Source: CAD feature listing. Evaluate the final solid. Frame: model axes, mm. Coordinates: 2 decimals unless noted, no trailing zeros. Loops run counter-clockwise (first coordinate to the right, second up) from the corner with the lowest first, then second, coordinate; pieces in that order, holes last. Notation, with made-up numbers: M 25,6 L 57,6 A17 cw 57,15 Z; hole C -27,5.25 d5. An arc over 180 degrees is marked long. Write each question's results on one line, items separated by ' | '. Start each with the question number.
from build123d import *

# Parameters (mm, degrees)
SKETCH_W        = 55
SKETCH_H        = 55
SKETCH_R        = 1.5
SKETCH_R_2      = 2.75
PAD_DEPTH       = 5
SKETCH001_R     = 4.5
POCKET_DEPTH    = 2
SKETCH002_R     = 3
POCKET001_DEPTH = 2


with BuildPart() as part:
    # Sketch → Pad (new body)
    with BuildSketch(Plane.XY):
        with Locations((27.5, 27.5)):
            Rectangle(SKETCH_W, SKETCH_H)
        with Locations((7.5, 47.5)):
            Circle(SKETCH_R, mode=Mode.SUBTRACT)
        with Locations((47.5, 7.5)):
            Circle(SKETCH_R, mode=Mode.SUBTRACT)
        with Locations((40, 40)):
            Circle(SKETCH_R_2, mode=Mode.SUBTRACT)
        with Locations((15, 15)):
            Circle(SKETCH_R_2, mode=Mode.SUBTRACT)
    extrude(amount=PAD_DEPTH)

    # Sketch001 → Pocket (cut)
    with BuildSketch(Plane.XY.offset(5)):
        with Locations((40, 40)):
            Circle(SKETCH001_R)
        with Locations((15, 15)):
            Circle(SKETCH001_R)
    extrude(amount=-POCKET_DEPTH, mode=Mode.SUBTRACT)

    # Sketch002 → Pocket001 (cut)
    with BuildSketch(Plane(origin=(0, 0, 0), x_dir=(1, 0, 0), z_dir=(0, 0, -1))):
        with Locations((47.5, -7.5)):
            Circle(SKETCH002_R)
        with Locations((7.5, -47.5)):
            Circle(SKETCH002_R)
    extrude(amount=-POCKET001_DEPTH, mode=Mode.SUBTRACT)


solid = part.part
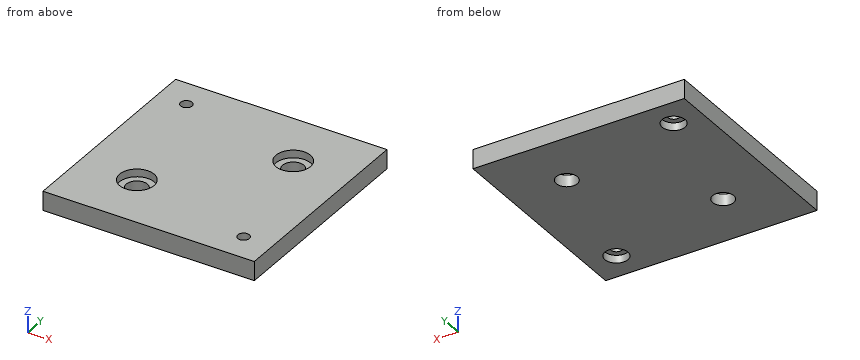
Item 1: Cut plane C-C (z = 1.3). Output: boundary loops of the cut face in (x, y).
Item 2: Cut plane A-A (x = 47.5). Output: boundary loops of the cut face in (y, z).
Item 3: Line query: probe 1 along X at (y, z) = (47.5, 1.05); probe 2 along Y at (x, z) = (40, 3.55); probe 3 along X at (y, z) = (47.5, 3.9). Output: solid intervals per line, ascending.
Item 4: Cut plane B-B (y = 40). Output: boundary loops of the cut face in (x, z).
Item 5: Cut plane D-D (x = 18.5). Output: boundary loops of the cut face in (y, z), then the cut area to 3 significant figures.
Item 6: First-contact query: pin 1 Ø8 at (x, y) = (40, 40) entering from +Z; pin 2 Ø3.5 at (x, y) = (7.5, 47.5) entering from -Z. Flat tips, straight axial feed; report the tip coordinate or a pass-through.
Response values:
1) outline: M 0,0 L 55,0 L 55,55 L 0,55 Z; hole C 7.5,47.5 d6; hole C 15,15 d5.5; hole C 40,40 d5.5; hole C 47.5,7.5 d6
2) outline: M 0,0 L 4.5,0 L 4.5,2 L 6,2 L 6,5 L 0,5 Z; M 9,2 L 10.5,2 L 10.5,0 L 55,0 L 55,5 L 9,5 Z
3) probe 1: x = 0 to 4.5, 10.5 to 55 | probe 2: y = 0 to 35.5, 44.5 to 55 | probe 3: x = 0 to 6, 9 to 55
4) outline: M 0,0 L 37.25,0 L 37.25,3 L 35.5,3 L 35.5,5 L 0,5 Z; M 42.75,0 L 55,0 L 55,5 L 44.5,5 L 44.5,3 L 42.75,3 Z
5) outline: M 0,0 L 55,0 L 55,5 L 17.83,5 L 17.83,3 L 12.17,3 L 12.17,5 L 0,5 Z | area: 264 mm2
6) pin 1: stops at z = 3 | pin 2: stops at z = 2
